Source: CAD feature listing. Evaluate the final solid. Frame: model axes, mm. A direction names the side the tool comes from. Give positions to 0.01 mm unless a question says otherwise; leave off trailing zeros. Order: outer loops, then holes, each group sorted by start corner. A loop starts at its lowest first (then second) coordinate and runs counter-clockwise, first axis right, second up. Notation, with made-up numbers: M 69.25,35 L 117.25,35 A25 ccw 117.25,58 Z; hole C 63.5,23 d11. An arc over 180 degrees is marked long. Answer in a Markdown table with one row per item. Add a question column.
(1) Mould query, pull axis X, two halves, no side actions, for faces 3 (the face through (-0.27, 3.52, 1.22)), 4 (the face through (-0.27, -1.48, 1.22)), 5 (the face through (0, -3, 0)). Classes: pulls with the +X half, pulls with the -X half, needs draft (parallel to the pull), parting line crosses it, or undercut.
(2) Material intervals for line 1 along X through (y, z) = (3.25, 0); line 2 along Y through (x, z) = (9, 8.5), sorted ascending.
(3) Pin query (flat end, axial travel): P1, Ø0.8, axis at x = -0.5, z = 0, coming from the +Y side; P2, Ø1.5, axis at x = -2.5, y = 0, coming from the -Z side; P3, Ø3, axis at x = 11, y = 3.5, coming from the +Z side. Return the tip coordinate at first contact, or that it passes through.
(4) Section query A-A, the plane x = 0. Return loops of the section in (y, z).
(5) Section query C-C, the plane z = 0. Return loops of the section in (x, y).
(6) Set-up query: faces 1 (the face through (-13.887, 2.535, 10.648)), 2 (the face through (0, 2, 0)). Return all of +Z, -Z, +X, -X, +Y, -Y with unobstructed straight access to the full face (end or side cutting, diameter ignored); none if empty.
(7) Section query B-B, the plane y = 4.5. Return loops of the section in (x, z).
(8) Section query D-D, the plane y = -1.75. Return loops of the section in (x, z), plus the area to 3 significant figures.
Autodesk Inventor part; units mm, degrees
ref_plane "YZ Plane" through (0, 0, 0) normal (1, 0, 0) x (0, 1, 0)
ref_plane "XZ Plane" through (0, 0, 0) normal (0, 1, 0) x (-1, 0, 0)
ref_plane "XY Plane" through (0, 0, 0) normal (0, 0, 1) x (1, 0, 0)
sketch "スケッチ1" plane through (0, 0, 0) normal (0, 1, 0) x (-1, 0, 0)
  circle A0 centre (0, 0) radius 12.5
  dimension "d0" = 25
extrude "押し出し1" add sketch "スケッチ1" along normal blind 5
sketch "スケッチ2" plane through (0, 5, 0) normal (0, 1, 0) x (1, 0, 0)
  circle A0 centre (0, 0) radius 12.5
  circle A1 centre (0, 0) radius 1.25
  dimension "d3" = 2.5
extrude "押し出し2" cut sketch "スケッチ2" against normal blind 3 contours A1
sketch "スケッチ3" plane through (0, 0, 0) normal (0, -1, 0) x (1, 0, 0)
  circle A0 centre (0, 0) radius 12.5
  circle A1 centre (0, 0) radius 1.25
  dimension "d6" = 2.5
extrude "押し出し3" add sketch "スケッチ3" along normal blind 3 contours A1
sketch "スケッチ4" plane through (0, 5, 0) normal (0, 1, 0) x (1, 0, 0)
  circle A0 centre (0, 0) radius 12.5
  circle A1 centre (0, 0) radius 17.5
  dimension "d9" = 35
extrude "押し出し4" add sketch "スケッチ4" against normal blind 5
properties part number "知能ロボコンシリンダ延長35mm"
Values follow:
| question | item | result |
|---|---|---|
| 1 | face 3 | undercut |
| 1 | face 4 | parting line crosses it |
| 1 | face 5 | needs draft |
| 2 | line 1 | x = -17.5 to -1.25, 1.25 to 17.5 |
| 2 | line 2 | y = 0 to 5 |
| 3 | P1 | stops at y = 2 |
| 3 | P2 | stops at z = -17.41 |
| 3 | P3 | stops at z = 14.7 |
| 4 | outline | M -3,-1.25 L 0,-1.25 L 0,-17.5 L 5,-17.5 L 5,-1.25 L 2,-1.25 L 2,1.25 L 5,1.25 L 5,17.5 L 0,17.5 L 0,1.25 L -3,1.25 Z |
| 5 | outline | M -17.5,0 L -1.25,0 L -1.25,-3 L 1.25,-3 L 1.25,0 L 17.5,0 L 17.5,5 L 1.25,5 L 1.25,2 L -1.25,2 L -1.25,5 L -17.5,5 Z |
| 6 | face 1 | +Y, -Y |
| 6 | face 2 | +Y |
| 7 | outline | C 0,0 d35; hole C 0,0 d2.5 |
| 8 | outline | C 0,0 d2.5 |
| 8 | area | 4.91 mm² |
